from build123d import *

# Parameters (mm, degrees)
SKETCH1_W           = 125
SKETCH1_H           = 125
BOSS_EXTRUDE1_DEPTH = 25
SKETCH2_W           = 102
SKETCH2_H           = 102
CUT_EXTRUDE1_DEPTH  = 15
SKETCH4_W           = 83.4
SKETCH4_H           = 11.5
SKETCH4_W_2         = 11.5
SKETCH4_H_2         = 83.4
CUT_EXTRUDE2_DEPTH  = 15
SKETCH5_W           = 9.3
SKETCH5_H           = 9.3
BOSS_EXTRUDE2_DEPTH = 8
CUT_EXTRUDE3_DEPTH  = 7


with BuildPart() as part:
    # Sketch1 → Boss-Extrude1 (new body)
    with BuildSketch(Plane(origin=(0, 0, 0), x_dir=(1, 0, 0), z_dir=(0, 1, 0))):
        with Locations((62.5, 62.5)):
            Rectangle(SKETCH1_W, SKETCH1_H)
    extrude(amount=BOSS_EXTRUDE1_DEPTH)

    # Sketch2 → Cut-Extrude1 (cut)
    with BuildSketch(Plane(origin=(0, 25, 0), x_dir=(1, 0, 0), z_dir=(0, 1, 0))):
        with Locations((62.5, 62.5)):
            Rectangle(SKETCH2_W, SKETCH2_H)
    extrude(amount=-CUT_EXTRUDE1_DEPTH, mode=Mode.SUBTRACT)

    # Sketch4 → Cut-Extrude2 (cut)
    with BuildSketch(Plane(origin=(0, 25, 0), x_dir=(1, 0, 0), z_dir=(0, 1, 0))):
        with Locations((62.5, 119.25)):
            Rectangle(SKETCH4_W, SKETCH4_H)
        with Locations((5.75, 62.5)):
            Rectangle(SKETCH4_W_2, SKETCH4_H_2)
        with Locations((62.5, 5.75)):
            Rectangle(SKETCH4_W, SKETCH4_H)
        with Locations((119.25, 62.5)):
            Rectangle(SKETCH4_W_2, SKETCH4_H_2)
    extrude(amount=-CUT_EXTRUDE2_DEPTH, mode=Mode.SUBTRACT)

    # Sketch5 → Boss-Extrude2 (add)
    with BuildSketch(Plane(origin=(0, 10, 0), x_dir=(1, 0, 0), z_dir=(0, 1, 0))):
        with Locations((108.85, 16.15)):
            Rectangle(SKETCH5_W, SKETCH5_H)
        with Locations((16.15, 16.15)):
            Rectangle(SKETCH5_W, SKETCH5_H)
        with Locations((16.15, 108.85)):
            Rectangle(SKETCH5_W, SKETCH5_H)
        with Locations((108.85, 108.85)):
            Rectangle(SKETCH5_W, SKETCH5_H)
    extrude(amount=BOSS_EXTRUDE2_DEPTH)

    # Sketch6 → Cut-Extrude3 (cut)
    with BuildSketch(Plane(origin=(0, 25, 0), x_dir=(1, 0, 0), z_dir=(0, 1, 0))):
        with BuildLine():
            Line((11.5, 11.5), (11.5, 16.5))
            ThreePointArc((11.5, 16.5), (9, 14), (11.5, 11.5))
        make_face()
        with BuildLine():
            Line((113.5, 11.5), (108.5, 11.5))
            ThreePointArc((108.5, 11.5), (111, 9), (113.5, 11.5))
        make_face()
        with BuildLine():
            Line((113.5, 108.5), (113.5, 113.5))
            ThreePointArc((113.5, 113.5), (116, 111), (113.5, 108.5))
        make_face()
        with BuildLine():
            Line((11.5, 113.5), (16.5, 113.5))
            ThreePointArc((16.5, 113.5), (14, 116), (11.5, 113.5))
        make_face()
    extrude(amount=-CUT_EXTRUDE3_DEPTH, mode=Mode.SUBTRACT)


solid = part.part
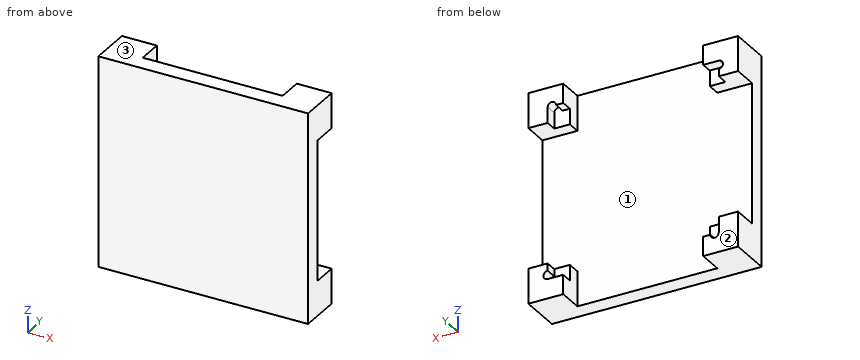
Geometry check sheet. Reference: the model listing, model coordinates, mm. Face numbers are marked on the shaded views. Give positions to 0.01 mm unless a question says otherwise; leave off trailing zeros. Loops run counter-clockwise (first coordinate to the right, second up) from the corner with the lowest first, then second, coordinate; pieces in that order, holes last. Notation, with made-up numbers: M -10.5,20 L 25.5,20 A28 cw 25.5,41 Z; hole C 1.25,-17.75 d7. An arc over 180 degrees is marked long. Answer as a JSON object with one key per item and string values. Group by question number.
Item 1: Sectioned sample at A-A on y = 11.5. Record the boundary of the cut face in (x, z), plus the area to 3 significant figures.
Item 2: Mould release check, pull along Z, two halves, no side actions. Record for the marked faces 1, 2 and 3: pulls with the +Z half, pulls with the -Z half, needs draft (parallel to the pull), parting line crosses it, or undercut.
Item 3: Sectioned sample at B-B on z = -14. Record the boundary of the cut face in (x, y), plus the area to 3 significant figures.
Item 4: Gauge pin test, flat ends, axial feed: pin 1 (4 mm diameter, centred on x = 42.5, z = -107.5, fed in from +Y); pin 2 (1.5 mm diameter, centred on x = 36, z = -47.5, fed in from -Y); pin 3 (10 mm diameter, centred on x = 30.5, y = 21.5, fed in from -Z); pin 4 (4.5 mm diameter, centred on x = 15, z = -15.5, fed in from +Y). Record the tip position at first contact, or that the pin passes through.
Item 5: Material ranges on L1, parallel to Y at x = 22, z = -98; L2, parallel to Y at x = 112.5, z = -18.5, recorded low to high.
Item 6: Sectioned sample at D-D on y = 21.25. Record the boundary of the cut face in (x, z).
Item 7: Sectioned sample at C-C on x = 48. Record the boundary of the cut face in (y, z), plus the area to 3 significant figures.
Findings below:
{
 "1": {"outline": "M 0,-125 L 20.8,-125 L 20.8,-104.2 L 0,-104.2 Z; M 0,-20.8 L 20.8,-20.8 L 20.8,0 L 0,0 Z; M 104.2,-125 L 125,-125 L 125,-104.2 L 104.2,-104.2 Z; M 104.2,-20.8 L 125,-20.8 L 125,0 L 104.2,0 Z", "area": "1,730 mm2"},
 "2": {"face 1": "undercut", "face 2": "needs draft", "face 3": "pulls with the +Z half"},
 "3": {"outline": "M 0,0 L 125,0 L 125,25 L 113.5,25 L 113.5,18 L 104.2,18 L 104.2,10 L 20.8,10 L 20.8,18 L 9,18 L 9,25 L 0,25 Z", "area": "1,730 mm2"},
 "4": {"pin 1": "y = 10", "pin 2": "y = 0", "pin 3": "through", "pin 4": "y = 18"},
 "5": {"L1": "0 to 10", "L2": "0 to 18"},
 "6": {"outline": "M 0,-125 L 20.8,-125 L 20.8,-113.5 L 16.5,-113.5 A2.5 cw 11.5,-113.5 L 11.5,-104.2 L 0,-104.2 Z; M 0,-20.8 L 11.5,-20.8 L 11.5,-16.5 A2.5 cw 11.5,-11.5 L 20.8,-11.5 L 20.8,0 L 0,0 Z; M 104.2,-125 L 125,-125 L 125,-104.2 L 113.5,-104.2 L 113.5,-108.5 A2.5 cw 113.5,-113.5 L 104.2,-113.5 Z; M 104.2,-11.5 L 108.5,-11.5 A2.5 cw 113.5,-11.5 L 113.5,-20.8 L 125,-20.8 L 125,0 L 104.2,0 Z"},
 "7": {"outline": "M 0,-125 L 10,-125 L 10,0 L 0,0 Z", "area": "1,250 mm2"}
}
